from build123d import *

# Parameters (mm, degrees)
SKETCH1_W           = 30.48
SKETCH1_H           = 22.86
SKETCH1_W_2         = 2.54
SKETCH1_H_2         = 12.7
BOSS_EXTRUDE2_DEPTH = 2.54
SKETCH3_R           = 1.016
BOSS_EXTRUDE3_DEPTH = 2.54
SKETCH4_W           = 30.48
SKETCH4_H           = 22.86
SKETCH4_W_2         = 2.54
SKETCH4_H_2         = 12.7
BOSS_EXTRUDE6_DEPTH = 2.54
SKETCH5_W           = 2.54
SKETCH5_H           = 12.7
BOSS_EXTRUDE7_DEPTH = 2.54
SKETCH6_W           = 12.669882096
SKETCH6_H           = 8.096264029
CUT_EXTRUDE1_DEPTH  = 0.762


with BuildPart() as part:
    # Sketch1 → Boss-Extrude2 (new body)
    with BuildSketch(Plane(origin=(0, 0, 0), x_dir=(1, 0, 0), z_dir=(0, 1, 0))):
        Rectangle(SKETCH1_W, SKETCH1_H)
        with Locations((-11.47489899, 0)):
            Rectangle(SKETCH1_W_2, SKETCH1_H_2, mode=Mode.SUBTRACT)
        with Locations((11.47489899, 0)):
            Rectangle(SKETCH1_W_2, SKETCH1_H_2, mode=Mode.SUBTRACT)
    extrude(amount=BOSS_EXTRUDE2_DEPTH)

    # Sketch3 → Boss-Extrude3 (add)
    with BuildSketch(Plane(origin=(0, 2.54, 0), x_dir=(1, 0, 0), z_dir=(0, 1, 0))):
        with Locations(Location((-5.318941048, 1.27, 0), (0, 0, 90))):
            Circle(SKETCH3_R)
        with Locations(Location((5.318941048, 1.27, 0), (0, 0, 90))):
            Circle(SKETCH3_R)
    extrude(amount=BOSS_EXTRUDE3_DEPTH)

    # Sketch4 → Boss-Extrude6 (add)
    with BuildSketch(Plane(origin=(0, 5.08, 0), x_dir=(1, 0, 0), z_dir=(0, 1, 0))):
        Rectangle(SKETCH4_W, SKETCH4_H)
        with Locations((-11.47489899, 0)):
            Rectangle(SKETCH4_W_2, SKETCH4_H_2, mode=Mode.SUBTRACT)
        with Locations((11.47489899, 0)):
            Rectangle(SKETCH4_W_2, SKETCH4_H_2, mode=Mode.SUBTRACT)
    extrude(amount=BOSS_EXTRUDE6_DEPTH)

    # Sketch5 → Boss-Extrude7 (add)
    with BuildSketch(Plane(origin=(0, 2.54, 0), x_dir=(1, 0, 0), z_dir=(0, 1, 0))):
        Polygon((-15.24, -11.43), (-15.24, 11.43), (15.24, 11.43), (15.24, -11.43), (8.89, -11.43), (8.89, 6.35), (-8.89, 6.35), (-8.89, -11.43), align=None)
        with Locations((-11.47489899, 0)):
            Rectangle(SKETCH5_W, SKETCH5_H, mode=Mode.SUBTRACT)
        with Locations((11.47489899, 0)):
            Rectangle(SKETCH5_W, SKETCH5_H, mode=Mode.SUBTRACT)
    extrude(amount=BOSS_EXTRUDE7_DEPTH)

    # Sketch6 → Cut-Extrude1 (cut)
    with BuildSketch(Plane(origin=(0, 2.54, 0), x_dir=(1, 0, 0), z_dir=(0, 1, 0))):
        with Locations((0, -5.167320683)):
            Rectangle(SKETCH6_W, SKETCH6_H)
    extrude(amount=-CUT_EXTRUDE1_DEPTH, mode=Mode.SUBTRACT)


solid = part.part
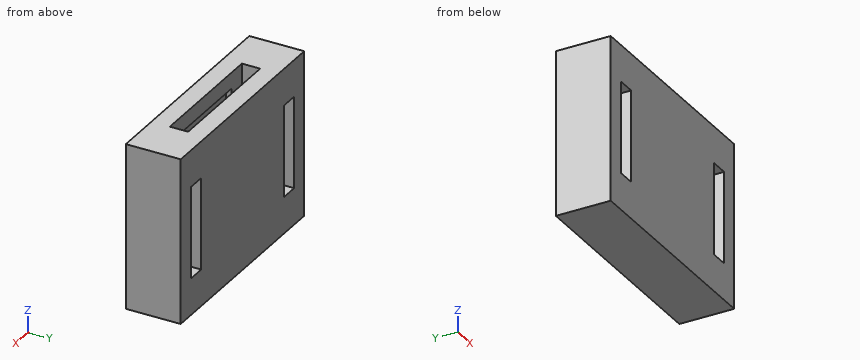
Part model, mm, in its own coordinate system. Round coordinates to 2 decimals unless told otherwise and drop trailing zeros. Order: outer loops, then holes, each group sorted by start corner. A loop starts at its lowest first (then second) coordinate and runs counter-clockwise, first axis right, second up. Notation, with made-up numbers: (-28, -39.75) -> (16, -39.75) arc R30 ccw to (16, -11.75) -> close; hole circle Ø3 at (-36, 43). An arc over 180 degrees is marked (long way). Put each result on its own line as item: value.
Q1. Pin check, flat tips, straight feed: pin 1 Ø8 at (x, z) = (-3.5, -4) entering from -Y; pin 2 Ø1.3 at (x, y) = (-2, 3.5) entering from +Z. Stop position of each tip, or through.
From the geometry:
pin 1: stops at y = 0
pin 2: stops at z = -6.35
Q2. Band-saw the part on B-B (z = -1.27). Give the cut face in (x, y), and give its area (3 significant figures).
From the geometry:
outline: (-15.24, 0) -> (-12.74, 0) -> (-12.74, 7.62) -> (-15.24, 7.62) -> close; (-10.2, 0) -> (10.2, 0) -> (10.2, 7.62) -> (-10.2, 7.62) -> close; (12.74, 0) -> (15.24, 0) -> (15.24, 7.62) -> (12.74, 7.62) -> close; hole (-8.89, 2.54) -> (-6.33, 2.54) -> (-6.33, 5.08) -> (-8.89, 5.08) -> close; hole (-4.3, 2.54) -> (4.3, 2.54) -> (4.3, 5.08) -> (-4.3, 5.08) -> close; hole (6.33, 2.54) -> (8.89, 2.54) -> (8.89, 5.08) -> (6.33, 5.08) -> close
area: 159 mm2
Q3. Band-saw the part on D-D (y = 0.5). Give the cut face in (x, z).
From the geometry:
outline: (-15.24, -11.43) -> (15.24, -11.43) -> (15.24, 11.43) -> (-15.24, 11.43) -> close; hole (-12.74, -6.35) -> (-10.2, -6.35) -> (-10.2, 6.35) -> (-12.74, 6.35) -> close; hole (10.2, -6.35) -> (12.74, -6.35) -> (12.74, 6.35) -> (10.2, 6.35) -> close
Q4. Band-saw the part on A-A (z = -4.5). Give the cut face in (x, y), and give its area (3 significant figures).
From the geometry:
outline: (-15.24, 0) -> (-12.74, 0) -> (-12.74, 7.62) -> (-15.24, 7.62) -> close; (-10.2, 0) -> (10.2, 0) -> (10.2, 7.62) -> (-10.2, 7.62) -> close; (12.74, 0) -> (15.24, 0) -> (15.24, 7.62) -> (12.74, 7.62) -> close; hole (-8.89, 2.54) -> (8.89, 2.54) -> (8.89, 5.08) -> (-8.89, 5.08) -> close
area: 148 mm2
Q5. Band-saw the part on C-C (x = -12). Give the cut face in (y, z), and give its area (3 significant figures).
From the geometry:
outline: (0, -11.43) -> (7.62, -11.43) -> (7.62, -6.35) -> (0, -6.35) -> close; (0, 6.35) -> (7.62, 6.35) -> (7.62, 11.43) -> (0, 11.43) -> close
area: 77.4 mm2
Q6. Wall check: line 1 (X direction, y = 3.75, z = -3.75); line 2 (X direction, y = 0.5, z = -5.75); line 3 (Y direction, x = -4, z = -5.5). Give the ranges that are in metal, low to high. Write a range as [from, to].
From the geometry:
line 1: x = [-15.24, -12.74], [-10.2, -8.89], [8.89, 10.2], [12.74, 15.24]
line 2: x = [-15.24, -12.74], [-10.2, 10.2], [12.74, 15.24]
line 3: y = [0, 2.54], [5.08, 7.62]
